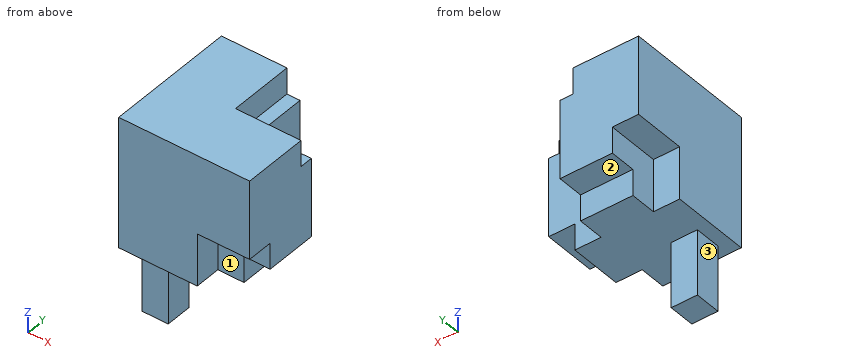
from build123d import *

# Parameters (mm, degrees)
F0_W      = 25.4
F0_H      = 25.4
F1_DEPTH  = 25.4
F2_W      = 10.16
F2_H      = 10.16
F3_DEPTH  = 5.08
F4_W      = 10.16
F4_H      = 10.16
F5_DEPTH  = 25.4
F6_W      = 5.08
F6_H      = 5.08
F7_DEPTH  = 12.7
F8_W      = 10.16
F8_H      = 10.16
F9_DEPTH  = 5.08
F10_W     = 5.08
F10_H     = 5.08
F11_DEPTH = 25.4
F12_W     = 5.08
F12_H     = 5.08
F13_DEPTH = 25.4
F14_W     = 12.7
F14_H     = 12.7
F15_DEPTH = 5.08


with BuildPart() as f1:
    # F0 (on Top) → F1 (new body)
    with BuildSketch(Plane.XY):
        with Locations((-12.7, -12.7)):
            Rectangle(F0_W, F0_H)
    extrude(amount=F1_DEPTH)

    # F2 (on face) → F3 (cut)
    with BuildSketch(Plane(origin=(-25.4, 0, 0), x_dir=(0, -1, 0), z_dir=(-1, 0, 0))):
        with Locations((5.08, 5.08)):
            Rectangle(F2_W, F2_H)
    extrude(amount=-F3_DEPTH, mode=Mode.SUBTRACT)

    # F4 (on face) → F5 (cut)
    with BuildSketch(Plane.XY.offset(25.4)):
        with Locations((-5.08, -5.08)):
            Rectangle(F4_W, F4_H)
    extrude(amount=-F5_DEPTH, mode=Mode.SUBTRACT)

    # F6 (on face) → F7 (join)
    with BuildSketch(Plane(origin=(0, 0, 0), x_dir=(1, 0, 0), z_dir=(0, 0, -1))):
        with Locations((-20.32, 20.32)):
            Rectangle(F6_W, F6_H)
    extrude(amount=F7_DEPTH)

    # F8 (on face) → F9 (cut)
    with BuildSketch(Plane.XZ.offset(25.4)):
        with Locations((-5.08, 5.08)):
            Rectangle(F8_W, F8_H)
    extrude(amount=-F9_DEPTH, mode=Mode.SUBTRACT)

    # F10 (on face) → F11 (cut)
    with BuildSketch(Plane.XZ.offset(20.32)):
        with Locations((-2.54, 2.54)):
            Rectangle(F10_W, F10_H)
    extrude(amount=-F11_DEPTH, mode=Mode.SUBTRACT)

    # F12 (on face) → F13 (cut)
    with BuildSketch(Plane(origin=(-20.32, 0, 0), x_dir=(0, -1, 0), z_dir=(-1, 0, 0))):
        with Locations((2.54, 2.54)):
            Rectangle(F12_W, F12_H)
    extrude(amount=-F13_DEPTH, mode=Mode.SUBTRACT)

    # F14 (on face) → F15 (cut)
    with BuildSketch(Plane.XY.offset(25.4)):
        with Locations((-6.35, -6.35)):
            Rectangle(F14_W, F14_H)
    extrude(amount=-F15_DEPTH, mode=Mode.SUBTRACT)


solid = f1.part
CAD build for the part. Positions are in the model's coordinates, mm. Face numbers are marked on the shaded views. A direction names the side the tool comes from. Give positions to 0.01 mm unless a question says otherwise; leave off trailing zeros. Loops run counter-clockwise (first coordinate to the right, second up) from the corner with the lowest first, then second, coordinate; pieces in that order, holes last. Notation, with made-up numbers: M 19.25,-28.75 L 69.25,-28.75 A36 ccw 69.25,5.25 Z; hole C 28.5,-18.5 d9. An arc over 180 degrees is marked long. Answer in a Markdown table with one row per item. Add a question column.
Item 1: Probe probe 1 along Z at (x, y) = (-14.5, -6); probe 2 along X at (y, z) = (-8, 2.5); probe 3 along Z at (x, y) = (-17, -4). List the from-to ranges inside material, lowest first.
Item 2: Drop flat-ended pins along their axis: P1, Ø10, axis at x = -15, y = -10, coming from the -Z side; P2, Ø2.5, axis at y = -15.5, z = 1.5, coming from the +X side; P3, Ø1.5, axis at x = -19.5, z = -7.5, coming from the +Y side; P4, Ø5, axis at x = -10.5, z = -3, coming from the +Y side. Give the stop position or say it passes through.
Item 3: Band-saw the part on A-A on y = -19.75. Give the cut face in (x, z), then the cut area to 3 significant figures.
Item 4: Band-saw the part on C-C on x = -22.25. Give the cut face in (y, z), then the cut area to 3 significant figures.
Item 5: Band-saw the part on B-B on z = 23.5. Give the cut face in (x, y).
Item 6: Tool access for the marked faces 1, 2 and 3: list every direction of +Z, -Z, +X, -X, +Y, -Y with a clear straight run to the whole face (end or side of a thin tool).
Item 7: Band-saw the part on D-D on y = -14.5. Give the cut face in (x, z).
Reply:
| question | item | result |
|---|---|---|
| 1 | probe 1 | z = 0 to 25.4 |
| 1 | probe 2 | x = -20.32 to -10.16 |
| 1 | probe 3 | z = 5.08 to 25.4 |
| 2 | P1 | stops at z = 0 |
| 2 | P2 | stops at x = -5.08 |
| 2 | P3 | stops at y = -17.78 |
| 2 | P4 | passes through |
| 3 | outline | M -25.4,0 L -22.86,0 L -22.86,-12.7 L -17.78,-12.7 L -17.78,0 L -5.08,0 L -5.08,5.08 L 0,5.08 L 0,25.4 L -25.4,25.4 Z |
| 3 | area | 684 mm^2 |
| 4 | outline | M -25.4,0 L -22.86,0 L -22.86,-12.7 L -17.78,-12.7 L -17.78,0 L -10.16,0 L -10.16,10.16 L 0,10.16 L 0,25.4 L -25.4,25.4 Z |
| 4 | area | 606 mm^2 |
| 5 | outline | M -25.4,-25.4 L 0,-25.4 L 0,-12.7 L -12.7,-12.7 L -12.7,0 L -25.4,0 Z |
| 6 | face 1 | -Z, +X, -Y |
| 6 | face 2 | -Z, +X, -X, +Y |
| 6 | face 3 | -Z, -X, +Y, -Y |
| 7 | outline | M -25.4,0 L -5.08,0 L -5.08,5.08 L 0,5.08 L 0,25.4 L -25.4,25.4 Z |
